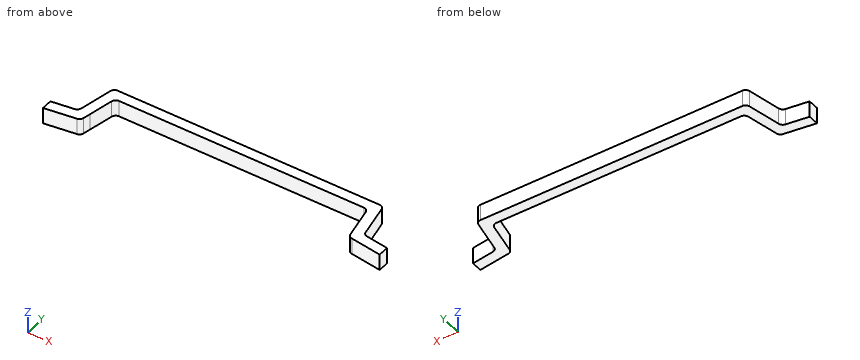
from build123d import *

# Parameters (mm, degrees)
BOSS_EXTRUDE1_DEPTH = 0.51
FILLET2_R           = 0.15
SKETCH3_W           = 0.51
SKETCH3_H           = 0.33
BOSS_EXTRUDE2_DEPTH = 3.8
MIRROR2_DEPTH       = 0.51


# Read off the part's stored shape, not the designer's step: Mirror2
with BuildPart() as part:
    # Sketch2 → Boss-Extrude1 (new body)
    with BuildSketch(Plane.XY):
        Polygon((0, 0.280138432), (0, 0), (0, -0.053104667), (1.080748407, 0.098784616), (1.148133843, 0.429247456), (1.327730115, 1.31), (1.515, 1.31), (1.515, 1.64), (1.058230308, 1.64), (0.803978227, 0.393130203), align=None)
    extrude(amount=BOSS_EXTRUDE1_DEPTH)

    # Fillet2
    fillet2_edges = [part.edges().sort_by_distance(p)[0] for p in [
        (1.080748407, 0.098784616, 0.255),
        (0.803978227, 0.393130203, 0.255),
        (1.058230308, 1.64, 0.255),
        (1.327730115, 1.31, 0.255),
    ]]
    fillet(fillet2_edges, radius=FILLET2_R)

    # Sketch3 → Boss-Extrude2 (add)
    with BuildSketch(Plane(origin=(1.515, 0, 0), x_dir=(0, 0, -1), z_dir=(1, 0, 0))):
        with Locations((-0.255, 1.475)):
            Rectangle(SKETCH3_W, SKETCH3_H)
    extrude(amount=BOSS_EXTRUDE2_DEPTH)

    # Mirror2 outline → Mirror2 (add)
    with BuildSketch(Plane.XY):
        with BuildLine():
            Line((5.315, 1.31), (9.179769973, 1.31))
            ThreePointArc((9.179769973, 1.31), (9.274650117, 1.276179852), (9.326745456, 1.189970108))
            Line((9.326745456, 1.189970108), (9.528080737, 0.202607957))
            ThreePointArc((9.528080737, 0.202607957), (9.572302902, 0.123299725), (9.654180255, 0.084037854))
            Line((9.654180255, 0.084037854), (10.63, -0.053104667))
            Line((10.63, -0.053104667), (10.63, 0.280138432))
            Line((10.63, 0.280138432), (9.930950436, 0.378383441))
            ThreePointArc((9.930950436, 0.378383441), (9.849073083, 0.417645311), (9.804850918, 0.496953543))
            Line((9.804850918, 0.496953543), (9.596245263, 1.519970108))
            ThreePointArc((9.596245263, 1.519970108), (9.544149925, 1.606179852), (9.44926978, 1.64))
            Line((9.44926978, 1.64), (5.315, 1.64))
            Line((5.315, 1.64), (5.315, 1.31))
        make_face()
    extrude(amount=MIRROR2_DEPTH)


solid = part.part
Read the model definition and answer for the solid it produces. Units are mm, in the model's axes. Give positions to 0.01 mm unless a question says otherwise; leave off trailing zeros. Loops run counter-clockwise (first coordinate to the right, second up) from the corner with the lowest first, then second, coordinate; pieces in that order, holes last. Notation, with made-up numbers: (55.25, 26.5) -> (86.25, 26.5) arc R29 ccw to (86.25, 65.5) -> close; hole circle Ø5 at (66, 38). An arc over 180 degrees is marked (long way). Use a Markdown table: item, result.
Q1. Section C-C, the plane x = 5.5 is taken. Determine the outline of the cut face in (y, z), then the cut area to 3 significant figures.
Solved:
| item | result |
|---|---|
| outline | (1.31, 0) -> (1.64, 0) -> (1.64, 0.51) -> (1.31, 0.51) -> close |
| area | 0.168 mm^2 |
Q2. Section A-A, the plane y = 0.6 is taken. Determine the outline of the cut face in (x, z).
Solved:
| item | result |
|---|---|
| outline | (0.85, 0) -> (1.18, 0) -> (1.18, 0.51) -> (0.85, 0.51) -> close; (9.45, 0) -> (9.78, 0) -> (9.78, 0.51) -> (9.45, 0.51) -> close |
Q3. Section B-B, the plane z = 0.15 is taken. Determine the outline of the cut face in (x, y).
Solved:
| item | result |
|---|---|
| outline | (0, -0.05) -> (0.98, 0.08) arc R0.15 ccw to (1.1, 0.2) -> (1.3, 1.19) arc R0.15 cw to (1.45, 1.31) -> (9.18, 1.31) arc R0.15 cw to (9.33, 1.19) -> (9.53, 0.2) arc R0.15 ccw to (9.65, 0.08) -> (10.63, -0.05) -> (10.63, 0.28) -> (9.93, 0.38) arc R0.15 cw to (9.8, 0.5) -> (9.6, 1.52) arc R0.15 ccw to (9.45, 1.64) -> (1.18, 1.64) arc R0.15 ccw to (1.03, 1.52) -> (0.83, 0.5) arc R0.15 cw to (0.7, 0.38) -> (0, 0.28) -> close |
Q4. Find the intervals of material crossed by line 1 along X through (y, z) = (0.2, 0.1); line 2 along Y through (x, z) = (4, 0.45); line 3 along X through (y, z) = (1, 0.35), in increasing order.
Solved:
| item | result |
|---|---|
| line 1 | x = 0 to 1.1, 9.53 to 10.63 |
| line 2 | y = 1.31 to 1.64 |
| line 3 | x = 0.93 to 1.26, 9.37 to 9.7 |
